Print and shaded views of the part. All mm, measured from the part's lowest x, y and z. A direction names the side the tool comes from. Give positions to 0.01 mm unless a question says otherwise; leave off trailing zeros. Order: outer loops, then holes, each group sorted by start corner. A loop starts at its lowest first (then second) coordinate and runs counter-clockwise, first axis right, second up. Notation, with made-up numbers: (-7.5, 17.5) -> (29.5, 17.5) arc R3 cw to (29.5, 21.5) -> close; hole circle Ø10 at (1.5, 21.5). An arc over 180 degrees is marked (long way). One line per question, with ' | ' between items. Start each with the question number.
(1) Which spindle directions (+Z, -Z, +X, -X, +Y, -Y) get a long thin tool onto all of the face, cutting with end or side? Do the marked faces 4 and 5. Say none if no direction does.
(2) Drill centre lines: L1, parallel to Y at x = 16, z = 22; L2, parallel to X at y = 60, z = 3; L3, parallel to Z at x = 36.5, y = 16. Where is each one in solid material? Low to high. Write a range as from..to.
(3) Cut at C-C (x = 37). Give the cut face in (y, z).
(4) Pin check, flat tips, straight feed: pin 1 Ø1 at (x, y) = (25.5, 64.5) entering from +Z; pin 2 Ø1.5 at (y, z) = (24, 25.5) entering from +X. Stop position of each tip, or through.
(5) Cut at D-D (y = 50). Give the cut face in (x, z).
(6) Cut at A-A (y = 22). Give the cut face in (x, z).
(7) Pull direction X, two halves, no side cores. Call the marked faces 1, 2 and 3: +X half, -X half, draft (parallel to the pull), parting line (faces both ways), or undercut.
(8) Cut at B-B (z = 15.5). Give the cut face in (x, y).
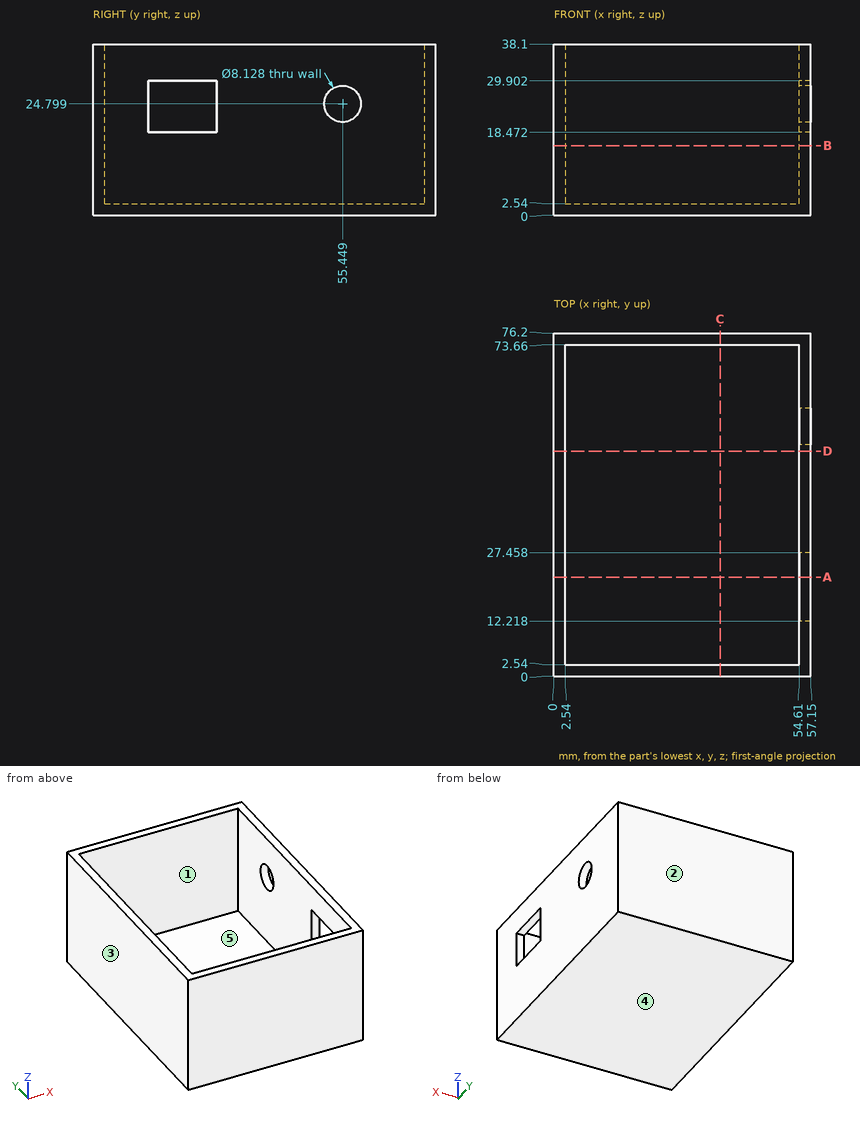
Result set:
1) face 4: -Z, +X, -X, +Y, -Y | face 5: +Z
2) L1: y = 0..2.54, 73.66..76.2 | L2: x = 0..2.54, 54.61..57.15 | L3: z = 0..2.54
3) outline: (0, 0) -> (76.2, 0) -> (76.2, 38.1) -> (73.66, 38.1) -> (73.66, 2.54) -> (2.54, 2.54) -> (2.54, 38.1) -> (0, 38.1) -> close
4) pin 1: stops at z = 2.54 | pin 2: stops at x = 2.54
5) outline: (0, 0) -> (57.15, 0) -> (57.15, 38.1) -> (54.61, 38.1) -> (54.61, 2.54) -> (2.54, 2.54) -> (2.54, 38.1) -> (0, 38.1) -> close
6) outline: (0, 0) -> (57.15, 0) -> (57.15, 18.47) -> (54.61, 18.47) -> (54.61, 2.54) -> (2.54, 2.54) -> (2.54, 38.1) -> (0, 38.1) -> close; (54.61, 29.9) -> (57.15, 29.9) -> (57.15, 38.1) -> (54.61, 38.1) -> close
7) face 1: undercut | face 2: draft | face 3: -X half
8) outline: (0, 0) -> (57.15, 0) -> (57.15, 76.2) -> (0, 76.2) -> close; hole (2.54, 2.54) -> (54.61, 2.54) -> (54.61, 73.66) -> (2.54, 73.66) -> close
